from build123d import *


with BuildPart() as part:
    # Эскиз1 → Повернуть1 (revolve)
    with BuildSketch(Plane.XY):
        Polygon((11.525952606, -1.221276852), (9.5, 0.804675754), (10.445620692, 1.750296446), (13, 1.750296446), (13, 1.395888621), (12.316457293, 1.395888621), (12.316457293, -0.208300549), (13, -0.208300549), (13, -0.785082607), (14.294407296, -0.785082607), (14.294407296, 1.750296446), (17, 1.750296446), (17, -1.654414722), (16.3705936, -2.283821122), (14.071003585, -2.283821122), (11.999272747, -3.593083063), (9.5, -3.293199519), align=None)
    revolve(axis=Axis((0, 17.208784833, 0), (0, -1, 0)))


solid = part.part
Read the model definition and answer for the solid it produces. Units are mm, in the model's axes. A direction names the side the tool comes from. Round coordinates to 2 decimals unless told otherwise and drop trailing zeros.
Q1. Consider probe 1 along X at (y, z) = (0.85, 3); probe 2 along X at (y, z) = (-0.3, 4); probe 3 along Z at (x, y) = (0, 0.55). Determine where each line is inside the solid, lowest interval first.
Q2. Determine the mould class of faces 1 (the face through (-10.316, 1.571, -7.91)), 2 (the face through (9.139, 0.024, 14.334)), 3 (the face through (4, 1.75, 14)), 4 (the face through (-3.099, 0.5, -13.954)) for opening direction X: released by +X, released by -X, zero draft, split by the parting line, or undercut.
Q3. Which of the six approach directions +Z, -Z, +X, -X, +Y, -Y give full straight-line access (tool end or side, diameter ignored) to faces 5 (the face through (-2.67, 0.583, -12.024)), 6 (the face through (4.8, -2.284, 13.4)), 7 (the face through (0, 1.75, 11)), 8 (the face through (-10.316, -0.501, -7.91))?
Q4. This flat-tipped pin is pushed along its axis until it touches: pin 1 (1 mm diameter, centred on x = 5, y = -0.5, fed in from +Z). Where does it stop, or does it pass through?
Output:
1. probe 1: x = -16.73 to -13.98, -11.95 to -9.06, 9.06 to 11.95, 13.98 to 16.73
1. probe 2: x = -16.52 to -13.72, -12.37 to -9.82, 9.82 to 12.37, 13.72 to 16.52
1. probe 3: z = -17 to -14.29, -12.32 to -9.75, 9.75 to 12.32, 14.29 to 17
2. face 1: undercut
2. face 2: split by the parting line
2. face 3: zero draft
2. face 4: undercut
3. face 5: none
3. face 6: -Y
3. face 7: +Z, -Z, +X, -X, +Y
3. face 8: +Y
4. pin 1: stops at z = 16.39
